Work out the finished part from the listing and answer in its coordinate system (mm). A direction names the side the tool comes from. Coordinates: 2 decimals unless noted, no trailing zeros. Order: outer loops, then holes, each group sorted by start corner. A loop starts at its lowest first (then second) coordinate and runs counter-clockwise, first axis right, second up.
1. The part is cut by section D-D, the plane y = 9. Give the vertices of the cut face in (x, z), then the cut area to 3 significant figures.
2. A tool of negligible diameter and unlimited length cuts with its end or side. For faces 4 (the cylindrical face through (94.69, 12.81, 10.61)), 5 (the flat face through (99.363, 7.846, 11.921)), 6 (the cylindrical face through (89.23, 5.5, 11.12)), from which of +Z, -Z, +X, -X, +Y, -Y can it reach the whole face along a straight path? Write none if from no direction.
3. Flat-ended cylindrical pins translate along their axes: pin 1 Ø1 at (y, z) = (2.5, 12) entering from -X; pin 2 Ø1.5 at (x, z) = (97, 11) entering from -Y; pin 3 Ø3 at (y, z) = (10, 9.5) entering from -X. Find the tip coordinate at first contact, or state that the pin passes through.
4. The part is cut by section A-A, the plane y = 7. Give the vertices of the cut face in (x, z).
5. The part is cut by section C-C, the plane z = 9.3. Give the vertices of the cut face in (x, y).
6. Find the intervals of material crossed by probe 1 along Y at (x, z) = (94, 8.5); probe 2 along Z at (x, y) = (97, 7.5); probe 3 along Y at (x, z) = (95.5, 11), in increasing order.
7. The part is cut by section B-B, the plane x = 94. Give the vertices of the cut face in (y, z).
8. Determine the mould class of faces 1 (the cylindrical face through (95.386, 6.425, 8.393)), 2 (the cylindrical face through (89.312, 10.499, 10.612)), 3 (the flat face through (98.084, 10.56, 11.921)) for opening direction X: +X half, -X half, draft (parallel to the pull), parting line (faces both ways), or undercut.
```python
from build123d import *

# Parameters (mm, degrees)
SKIZZE2_R                       = 5
AUFSATZ_LINEAR_AUSTRAGEN1_DEPTH = 1
SKIZZE2_4_R                     = 5.85
SKIZZE2_4_R_2                   = 5
AUFSATZ_LINEAR_AUSTRAGEN2_DEPTH = 5.5
SKIZZE3_R                       = 0.4
AUFSATZ_LINEAR_AUSTRAGEN3_DEPTH = 5.5
KREISMUSTER1_COUNT              = 6
SCHNITT_LINEAR_AUSTRAGEN1_DEPTH = 3
SKIZZE5_R                       = 1.5
SCHNITT_LINEAR_AUSTRAGEN2_DEPTH = 102.03637778


with BuildPart() as part:
    # Skizze2 → Aufsatz-Linear austragen1 (new body)
    with BuildSketch(Plane.XY.offset(7.9)):
        with Locations((94, 7)):
            Circle(SKIZZE2_R)
    extrude(amount=AUFSATZ_LINEAR_AUSTRAGEN1_DEPTH)

    # Skizze2<4> → Aufsatz-Linear austragen2 (add)
    with BuildSketch(Plane.XY.offset(7.9)):
        with Locations(Location((94, 7, 0), (0, 0, 180))):
            Circle(SKIZZE2_4_R)
        with Locations(Location((94, 7, 0), (0, 0, 180))):
            Circle(SKIZZE2_4_R_2, mode=Mode.SUBTRACT)
    extrude(amount=AUFSATZ_LINEAR_AUSTRAGEN2_DEPTH)

    # Skizze3 → Aufsatz-Linear austragen3 (add)
    with BuildSketch(Plane.XY.offset(7.9)):
        with Locations((91.714816695, 12.22187105)):
            Circle(SKIZZE3_R)
    aufsatz_linear_austragen3 = extrude(amount=AUFSATZ_LINEAR_AUSTRAGEN3_DEPTH)

    # Kreismuster1: Aufsatz-Linear austragen3 ×6 about axis
    kreismuster1_axis = Axis((94, 7, 0), (0, 0, 1))
    for i in range(1, KREISMUSTER1_COUNT):
        add(aufsatz_linear_austragen3.rotate(kreismuster1_axis, i * 360 / KREISMUSTER1_COUNT))

    # Skizze4 → Schnitt-Linear austragen1 (cut)
    with BuildSketch(Plane.XY.offset(13.4)):
        Polygon((93.366072607, 8.359461681), (100.290761443, 11.588497115), (101.558616228, 8.869573754), (94.633927393, 5.640538319), align=None)
    extrude(amount=-SCHNITT_LINEAR_AUSTRAGEN1_DEPTH, mode=Mode.SUBTRACT)

    # Skizze5 → Schnitt-Linear austragen2 (cut, through all)
    with BuildSketch(Plane.XY.offset(7.9)):
        with Locations((94, 7)):
            Circle(SKIZZE5_R)
    extrude(amount=SCHNITT_LINEAR_AUSTRAGEN2_DEPTH, mode=Mode.SUBTRACT)


solid = part.part
```
Geometry says:
1. outline: (88.5, 7.9) - (99.5, 7.9) - (99.5, 10.4) - (98.58, 10.4) - (98.58, 8.9) - (89.42, 8.9) - (89.42, 13.4) - (88.5, 13.4) - close
1. area: 16.5 mm2
2. face 4: +Z, -Z, +Y
2. face 5: +Z, +Y
2. face 6: +Z
3. pin 1: stops at x = 89.73
3. pin 2: stops at y = 1.38
3. pin 3: stops at x = 88.35
4. outline: (88.15, 7.9) - (92.5, 7.9) - (92.5, 8.9) - (89, 8.9) - (89, 13.4) - (88.15, 13.4) - close; (95.5, 7.9) - (99.85, 7.9) - (99.85, 13.4) - (99, 13.4) - (99, 8.9) - (95.5, 8.9) - close
5. outline: (88.16, 7.27) arc R5.85 ccw to (90.24, 2.52) arc R0.4 ccw to (90.84, 2.08) arc R5.85 ccw to (96, 1.5) arc R0.4 ccw to (96.68, 1.8) arc R5.85 ccw to (99.76, 5.98) arc R0.4 ccw to (99.84, 6.73) arc R5.85 ccw to (97.76, 11.48) arc R0.4 ccw to (97.16, 11.92) arc R5.85 ccw to (92, 12.5) arc R0.4 ccw to (91.32, 12.2) arc R5.85 ccw to (88.24, 8.02) arc R0.4 ccw to start; hole circle Ø10 at (94, 7)
6. probe 1: y = 1.15 to 5.5, 8.5 to 12.85
6. probe 2: z = 7.9 to 8.9
6. probe 3: y = 1.35 to 2.23, 11.77 to 12.65
7. outline: (1.15, 7.9) - (5.5, 7.9) - (5.5, 8.9) - (2, 8.9) - (2, 13.4) - (1.15, 13.4) - close; (8.5, 7.9) - (12.85, 7.9) - (12.85, 13.4) - (12, 13.4) - (12, 8.9) - (8.5, 8.9) - close
8. face 1: undercut
8. face 2: -X half
8. face 3: +X half
